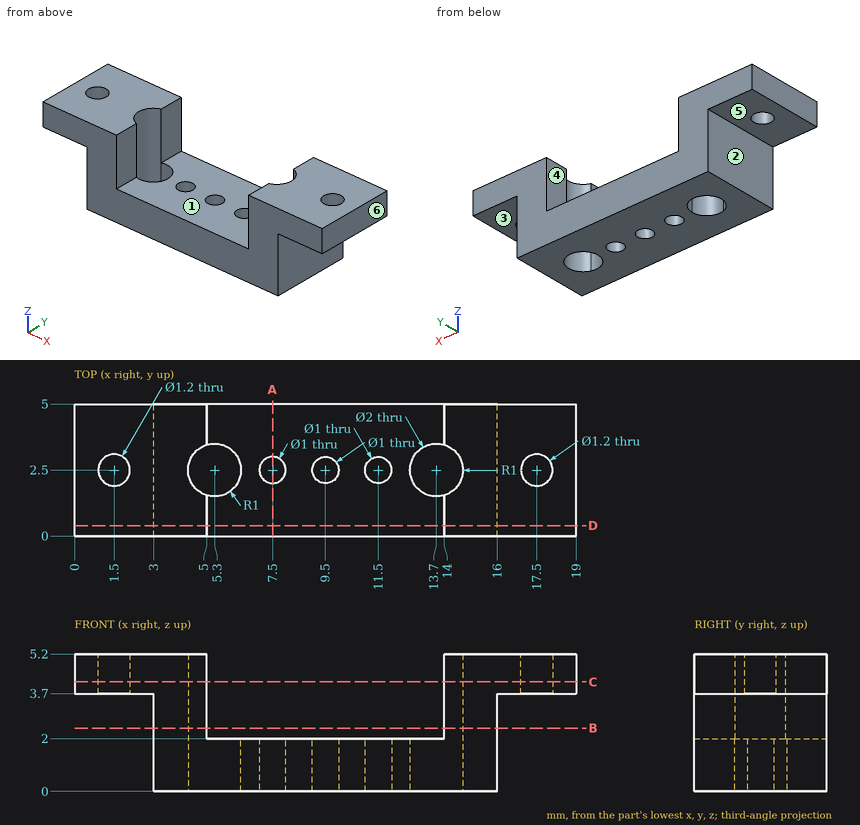
The figure shows three views and two pictorial views of one solid part (mm, origin at its lowest corner). Answer the questions. A direction names the side the tool comes from. Give positions to 0.01 mm unless a question says otherwise; leave off trailing zeros. Write each loop counter-clockwise with the first axis right and the second up, starting at its lowest first coordinate (ties: lowest second). Pieces come first, ordered by that corner, then holes.
Q1. The part is cut by section B-B on z = 2.4. Give the vertices of the cut face in (x, y), and give its area (3 significant figures).
Answer:
outline: (3, 0) - (5, 0) - (5, 1.55) arc R1 cw to (5, 3.45) - (5, 5) - (3, 5) - close; (14, 0) - (16, 0) - (16, 5) - (14, 5) - (14, 3.45) arc R1 cw to (14, 1.55) - close
area: 18.0 mm2
Q2. Given pin 1 (1.7 mm diameter, centred on y = 4.5, z = 3.5, fed in from -X); pin 2 (0.7 mm diameter, centred on x = 17.5, y = 2.5, fed in from +Z); pin 3 (0.9 mm diameter, centred on x = 1, y = 2, fed in from -Z); pin 4 (1.1 mm diameter, centred on y = 2.5, z = 1.5, fed in from +X), each flat-ended and moving along its own axis, determine where each tip first touches the part or whether it passes through.
Answer:
pin 1: stops at x = 0
pin 2: passes through
pin 3: stops at z = 3.7
pin 4: stops at x = 16
Q3. For a pull along X with two mould halves and no side action, classify the marked faces 4, 5 and 6 as released by +X, released by -X, zero draft, split by the parting line, or undercut.
Answer:
face 4: undercut
face 5: zero draft
face 6: released by +X
Q4. Straight lines are drawn through the part: L1, parallel to X at y = 4.6, z = 5; L2, parallel to X at y = 2.35, z = 4.8; L3, parallel to Y at x = 9.5, z = 1.15. For each, find the intervals that lie inside material, in ascending order.
Answer:
L1: x = 0 to 5, 14 to 19
L2: x = 0 to 0.92, 2.08 to 4.31, 14.69 to 16.92, 18.08 to 19
L3: y = 0 to 2, 3 to 5
Q5. The part is cut by section C-C on z = 4.15. Give the vertices of the cut face in (x, y).
Answer:
outline: (0, 0) - (5, 0) - (5, 1.55) arc R1 cw to (5, 3.45) - (5, 5) - (0, 5) - close; (14, 0) - (19, 0) - (19, 5) - (14, 5) - (14, 3.45) arc R1 cw to (14, 1.55) - close; hole circle Ø1.2 at (1.5, 2.5); hole circle Ø1.2 at (17.5, 2.5)
Q6. The part is cut by section D-D on y = 0.4. Give the vertices of the cut face in (x, z), and give its area (3 significant figures).
Answer:
outline: (0, 3.7) - (3, 3.7) - (3, 0) - (16, 0) - (16, 3.7) - (19, 3.7) - (19, 5.2) - (14, 5.2) - (14, 2) - (5, 2) - (5, 5.2) - (0, 5.2) - close
area: 47.8 mm2
Q7. The part is cut by section A-A on x = 7.5. Give the vertices of the cut face in (y, z), and give its area (3 significant figures).
Answer:
outline: (0, 0) - (2, 0) - (2, 2) - (0, 2) - close; (3, 0) - (5, 0) - (5, 2) - (3, 2) - close
area: 8.00 mm2
Q8. A tool of negligible diameter and unlimited length cuts with its end or side. For the marked faces 1, 2 and 3, from which of +Z, -Z, +X, -X, +Y, -Y can it reach the whole face along a straight path? Write none if from no direction.
Answer:
face 1: +Z, +Y, -Y
face 2: -Z, -X, +Y, -Y
face 3: -Z, +X, +Y, -Y
